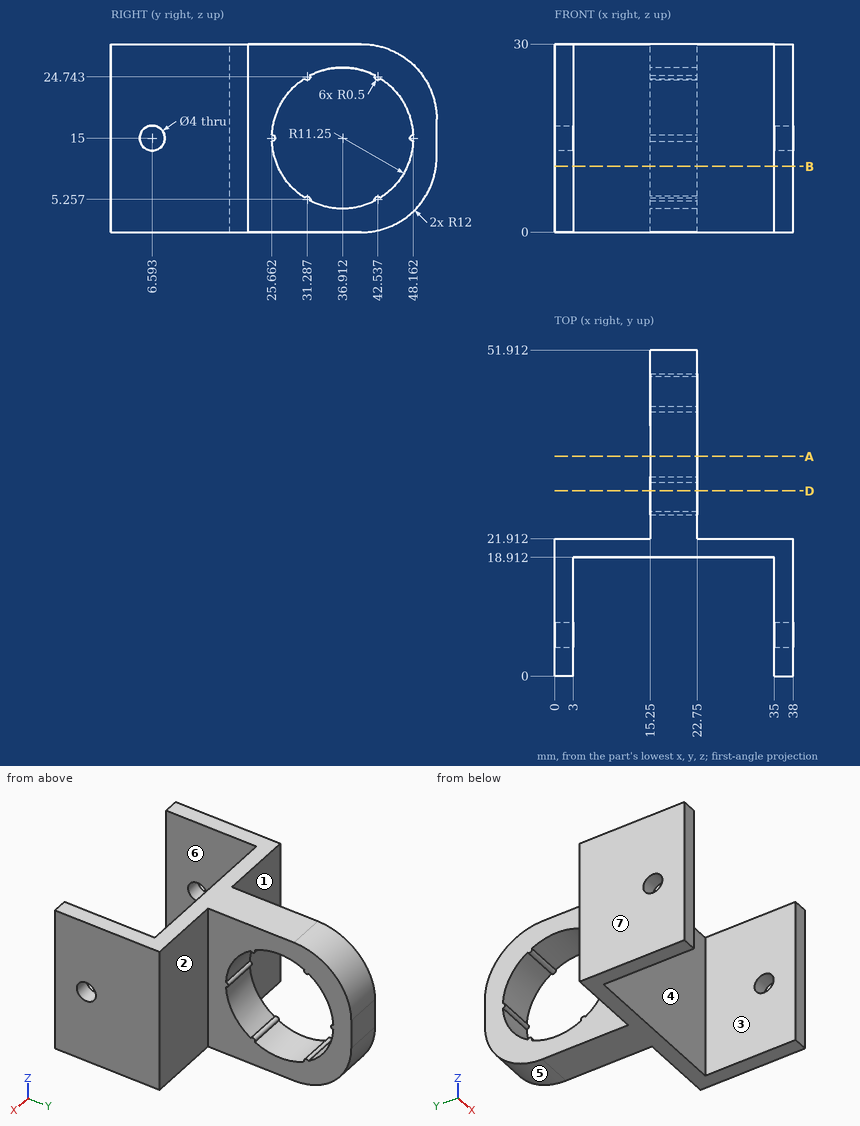
Verification items for this drawing (mm, ordinates from the low corner). A direction names the side the tool comes from. Give positions to 0.01 mm unless a question says otherwise; leave off trailing zeros. Loops run counter-clockwise (first coordinate to the right, second up) from the corner with the lowest first, then second, coordinate; pieces in that order, holes last.
1. Cross-section at A-A on y = 35. Record the cut outline in (x, z), and give its area (3 significant figures).
Derived:
outline: (15.25, 0) - (22.75, 0) - (22.75, 3.91) - (15.25, 3.91) - close; (15.25, 26.09) - (22.75, 26.09) - (22.75, 30) - (15.25, 30) - close
area: 58.7 mm2
2. Material ranges on probe 1 along Y at (x, z) = (36.3, 15); probe 2 along X at (y, z) = (15, 24.5); probe 3 along X at (y, z) = (47, 9.5), recorded low to high.
Derived:
probe 1: y = 0 to 4.59, 8.59 to 21.91
probe 2: x = 0 to 3, 35 to 38
probe 3: x = 15.25 to 22.75
3. Tool access check on the marked faces 1, 2 and 3. Record the directions out of +Z, -Z, +X, -X, +Y, -Y that give a thin tool (end or side, any length) a straight path to the whole face; none if there is none.
Derived:
face 1: +Z, -Z, -X, +Y
face 2: +Z, -Z, +X, +Y
face 3: +Z, -Z, -Y
4. Cross-section at D-D on y = 29.5. Record the cut outline in (x, z).
Derived:
outline: (15.25, 0) - (22.75, 0) - (22.75, 6.54) - (15.25, 6.54) - close; (15.25, 23.46) - (22.75, 23.46) - (22.75, 30) - (15.25, 30) - close
5. Go/stop test with flat-tipped pins: P1, Ø8, axis at x = 20, y = 46, coming from the +Z side; P2, Ø1.5, axis at x = 7.5, z = 7, coming from the +Y side; P3, Ø15, axis at x = 12, z = 15, coming from the -Y side. Record where each tip stops, or that it passes through.
Derived:
P1: stops at z = 29.82
P2: stops at y = 21.91
P3: stops at y = 18.91
6. Cross-section at B-B on z = 10.5. Record the cut outline in (x, y), and give its area (3 significant figures).
Derived:
outline: (0, 0) - (3, 0) - (3, 18.91) - (35, 18.91) - (35, 0) - (38, 0) - (38, 21.91) - (22.75, 21.91) - (22.75, 26.6) - (15.25, 26.6) - (15.25, 21.91) - (0, 21.91) - close; (15.25, 47.22) - (22.75, 47.22) - (22.75, 51.82) - (15.25, 51.82) - close
area: 297 mm2
7. Release check for a two-part mould opening along X. For the marked faces 4, 5, 6 and 7 record: +X half, -X half, draft (parallel to the pull), parting line (faces both ways), or undercut.
Derived:
face 4: undercut
face 5: draft
face 6: undercut
face 7: -X half
